from build123d import *

# Parameters (mm, degrees)
SKETCH1_W           = 133.35
SKETCH1_H           = 44.958
BOSS_EXTRUDE1_DEPTH = 2.54
CUT_EXTRUDE1_DEPTH  = 141.747631824
SKETCH6_R           = 3.81
CUT_EXTRUDE3_DEPTH  = 141.747631824
SKETCH7_W           = 2.54
SKETCH7_H           = 5.08
BOSS_EXTRUDE2_DEPTH = 4.572
SKETCH9_R           = 0.762
CUT_EXTRUDE4_DEPTH  = 110.343091103
FILLET2_R           = 2.54
FILLET3_R           = 2.54
FILLET4_R           = 1.27
SKETCH16_R          = 1.4986
CUT_EXTRUDE8_DEPTH  = 2.032
SKETCH17_R          = 1.524
CUT_EXTRUDE9_DEPTH  = 2.032


with BuildPart() as part:
    # Sketch1 → Boss-Extrude1 (new body)
    with BuildSketch(Plane(origin=(0, 0, 0), x_dir=(1, 0, 0), z_dir=(0, 1, 0))):
        with Locations((66.675, -22.479)):
            Rectangle(SKETCH1_W, SKETCH1_H)
    extrude(amount=BOSS_EXTRUDE1_DEPTH)

    # Sketch2 → Cut-Extrude1 (cut, through all)
    with BuildSketch(Plane(origin=(133.35, 0, 0), x_dir=(0, 0, -1), z_dir=(1, 0, 0))):
        Polygon((-44.958, 0), (-44.958, 2.54), (-42.418, 2.54), align=None)
    extrude(amount=-CUT_EXTRUDE1_DEPTH, mode=Mode.SUBTRACT)

    # Sketch6 → Cut-Extrude3 (cut, through all)
    with BuildSketch(Plane(origin=(0, 2.54, 0), x_dir=(1, 0, 0), z_dir=(0, 1, 0))):
        with Locations(Location((27.94, -26.924, 0), (0, 0, 270))):
            Circle(SKETCH6_R)
    extrude(amount=-CUT_EXTRUDE3_DEPTH, mode=Mode.SUBTRACT)

    # Sketch7 → Boss-Extrude2 (add)
    with BuildSketch(Plane.XZ):
        with Locations((100.838, 25.4)):
            Rectangle(SKETCH7_W, SKETCH7_H)
    extrude(amount=BOSS_EXTRUDE2_DEPTH)

    # Sketch9 → Cut-Extrude4 (cut, through all)
    with BuildSketch(Plane.ZY.offset(-99.568)):
        with Locations((25.4, -2.286)):
            Circle(SKETCH9_R)
    extrude(amount=-CUT_EXTRUDE4_DEPTH, mode=Mode.SUBTRACT)

    # Fillet2
    fillet2_edges = [part.edges().sort_by_distance(p)[0] for p in [
        (100.838, -4.572, 27.94),
    ]]
    fillet(fillet2_edges, radius=FILLET2_R)

    # Fillet3
    fillet3_edges = [part.edges().sort_by_distance(p)[0] for p in [
        (100.838, -4.572, 22.86),
    ]]
    fillet(fillet3_edges, radius=FILLET3_R - 0.0001)  # a hair under: the kernel refuses the full size

    # Fillet4
    fillet4_edges = [part.edges().sort_by_distance(p)[0] for p in [
        (66.675, 0, 0),
        (66.675, 2.54, 0),
    ]]
    fillet(fillet4_edges, radius=FILLET4_R - 0.0001)  # a hair under: the kernel refuses the full size

    # Sketch16 → Cut-Extrude8 (cut)
    with BuildSketch(Plane.XZ):
        with Locations(Location((20.955, 5.9436, 0), (0, 0, 270))):
            Circle(SKETCH16_R)
        with Locations(Location((30.9626, 5.9436, 0), (0, 0, 270))):
            Circle(SKETCH16_R)
        with Locations(Location((102.3874, 5.9436, 0), (0, 0, 270))):
            Circle(SKETCH16_R)
        with Locations(Location((112.395, 5.9436, 0), (0, 0, 270))):
            Circle(SKETCH16_R)
    extrude(amount=-CUT_EXTRUDE8_DEPTH, mode=Mode.SUBTRACT)

    # Sketch17 → Cut-Extrude9 (cut)
    with BuildSketch(Plane(origin=(0, 0, 0), x_dir=(1, 0, 0), z_dir=(0, 1, 0))):
        with Locations(Location((38.1, -16.764, 0), (0, 0, 270))):
            Circle(SKETCH17_R)
        with Locations(Location((17.78, -16.764, 0), (0, 0, 270))):
            Circle(SKETCH17_R)
    extrude(amount=CUT_EXTRUDE9_DEPTH, mode=Mode.SUBTRACT)


solid = part.part
Source: CAD feature listing. Evaluate the final solid. Frame: model axes, mm. A direction names the side the tool comes from. Give positions to 0.01 mm unless a question says otherwise; leave off trailing zeros. Write each loop counter-clockwise with the first axis right and the second up, starting at its lowest first coordinate (ties: lowest second). Pieces come first, ordered by that corner, then holes. Notation, with made-up numbers: M -21.75,0.25 L 2.25,0.25 A22 cw 2.25,17.25 Z; hole C 36,37 d2. An arc over 180 degrees is marked long. Return JSON: item names as keys, results as strings. Group by question number.
1) Material intervals for line 1 along X through (y, z) = (0.5, 7); line 2 along X through (y, z) = (-1.75, 23); line 3 along X through (y, z) = (2, 26.5), sorted ascending. Write a range as [from, to].
2) Cut plane B-B, the plane z = 35. Output: boundary loops of the cut face in (x, y).
3) Pull-direction query (X, two-part tool) for faces 1 (the face through (112, 2.032, 6)), 2 (the face through (66, 2.54, 22)), 3 (the face through (102.108, -1, 25)); classes: pulls with the +X half, pulls with the -X half, needs draft (parallel to the pull), parting line crosses it, or undercut.
4) Set-up query: faces 4 (the face through (26.481, 1.288, 30.443)), 5 (the face through (21, 2.032, 6)). Return all of +Z, -Z, +X, -X, +Y, -Y with unobstructed straight access to the full face (end or side cutting, diameter ignored); none if empty.
5) Pin query (flat end, axial travel): P1, Ø22, axis at x = 39, z = 16, coming from the -Y side; P2, Ø0.9, axis at x = 112.5, z = 5.5, coming from the -Y side; P3, Ø2, axis at y = -2.286, z = 25.4, coming from the -X side. Return the tip coordinate at first contact, or that it passes through.
Recorded:
{
 "1": {"line 1": "x = [0, 19.89], [22.02, 29.9], [32.03, 101.32], [103.45, 111.33], [113.46, 133.35]", "line 2": "x = [99.57, 102.11]", "line 3": "x = [0, 24.15], [31.73, 133.35]"},
 "2": {"outline": "M 0,0 L 133.35,0 L 133.35,2.54 L 0,2.54 Z"},
 "3": {"face 1": "undercut", "face 2": "needs draft", "face 3": "pulls with the +X half"},
 "4": {"face 4": "+Y, -Y", "face 5": "-Y"},
 "5": {"P1": "stops at y = 0", "P2": "stops at y = 2.03", "P3": "stops at x = 99.57"}
}
